from build123d import *

# Parameters (mm, degrees)
SKETCH_1_W          = 26.42
SKETCH_1_H          = 6.6
EXTRUDE_1_DEPTH     = 4.4
SKETCH_2_W          = 12.3
SKETCH_2_H          = 8.6
EXTRUDE_2_DEPTH     = 1.6
SKETCH_3_W          = 4.1
SKETCH_3_H          = 6.6
EXTRUDE_3_DEPTH     = 9.7
FILLET_1_R          = 3
FILLET_2_R          = 1
SKETCH_4_W          = 6
SKETCH_4_H          = 1
EXTRUDE_4_DEPTH     = 1
SKETCH_5_W          = 0.293200104
SKETCH_5_H          = 0.293200104
SKETCH_5_W_2        = 0.377208019
SKETCH_5_W_3        = 0.433090687
EXTRUDE_5_DEPTH     = 1
SKETCH_6_W          = 0.293200104
SKETCH_6_H          = 0.267980564
SKETCH_6_W_2        = 0.377208019
SKETCH_6_W_3        = 0.433090687
EXTRUDE_6_DEPTH     = 6
SKETCH_7_R          = 1.75
CUT_EXTRUDE_1_DEPTH = 6


with BuildPart() as part:
    # 草图1 → 凸台-拉伸1 (new body)
    with BuildSketch(Plane(origin=(0, 0, 0), x_dir=(1, 0, 0), z_dir=(0, 1, 0))):
        with Locations((13.21, 3.3)):
            Rectangle(SKETCH_1_W, SKETCH_1_H)
    extrude(amount=EXTRUDE_1_DEPTH)

    # 草图2 → 凸台-拉伸2 (add)
    with BuildSketch(Plane(origin=(0, 0, 0), x_dir=(-1, 0, 0), z_dir=(0, -1, 0))):
        with Locations((-13.21, -4.3)):
            Rectangle(SKETCH_2_W, SKETCH_2_H)
    extrude(amount=-EXTRUDE_2_DEPTH)

    # 草图3 → 凸台-拉伸3 (add)
    with BuildSketch(Plane(origin=(0, 4.4, 0), x_dir=(1, 0, 0), z_dir=(0, 1, 0))):
        with Locations((8.21, 3.3)):
            Rectangle(SKETCH_3_W, SKETCH_3_H)
        with Locations((18.21, 3.3)):
            Rectangle(SKETCH_3_W, SKETCH_3_H)
    extrude(amount=EXTRUDE_3_DEPTH)

    # 圆角1
    fillet_1_edges = [part.edges().sort_by_distance(p)[0] for p in [
        (0, 2.2, -6.6),
        (26.42, 2.2, -6.6),
        (26.42, 2.2, 0),
        (0, 2.2, 0),
    ]]
    fillet(fillet_1_edges, radius=FILLET_1_R)

    # 圆角2
    fillet_2_edges = [part.edges().sort_by_distance(p)[0] for p in [
        (7.06, 0.8, 8.6),
        (19.36, 0.8, 8.6),
    ]]
    fillet(fillet_2_edges, radius=FILLET_2_R)

    # 草图4 → 凸台-拉伸4 (add)
    with BuildSketch(Plane(origin=(0, 0, 0), x_dir=(-1, 0, 0), z_dir=(0, -1, 0))):
        with Locations((-13.21, -7.5)):
            Rectangle(SKETCH_4_W, SKETCH_4_H)
    extrude(amount=EXTRUDE_4_DEPTH)

    # 草图5 → 凸台-拉伸5 (add)
    with BuildSketch(Plane(origin=(0, -1, 0), x_dir=(-1, 0, 0), z_dir=(0, -1, 0))):
        with Locations((-11.206465954, -7.438185624)):
            Rectangle(SKETCH_5_W, SKETCH_5_H)
        with Locations((-13.359332723, -7.438185624)):
            Rectangle(SKETCH_5_W_2, SKETCH_5_H)
        with Locations((-15.259343482, -7.438185624)):
            Rectangle(SKETCH_5_W_3, SKETCH_5_H)
    extrude(amount=EXTRUDE_5_DEPTH)

    # 草图6 → 凸台-拉伸6 (add)
    with BuildSketch(Plane.XY.offset(7.584785676)):
        with Locations((11.206465954, -1.866009718)):
            Rectangle(SKETCH_6_W, SKETCH_6_H)
        with Locations((13.359332723, -1.866009718)):
            Rectangle(SKETCH_6_W_2, SKETCH_6_H)
        with Locations((15.259343482, -1.866009718)):
            Rectangle(SKETCH_6_W_3, SKETCH_6_H)
    extrude(amount=EXTRUDE_6_DEPTH)

    # 草图7 → 切除-拉伸1 (cut)
    with BuildSketch(Plane(origin=(0, 4.4, 0), x_dir=(1, 0, 0), z_dir=(0, 1, 0))):
        with Locations(Location((2.8, 3.3, 0), (0, 0, 270))):
            Circle(SKETCH_7_R)
        with Locations(Location((23.62, 3.3, 0), (0, 0, 270))):
            Circle(SKETCH_7_R)
    extrude(amount=-CUT_EXTRUDE_1_DEPTH, mode=Mode.SUBTRACT)


solid = part.part
Part model, mm, in its own coordinate system. A direction names the side the tool comes from. Coordinates: 2 decimals unless noted, no trailing zeros. Loops run counter-clockwise (first coordinate to the right, second up) from the corner with the lowest first, then second, coordinate; pieces in that order, holes last. Notation, with made-up numbers: M -14,34.25 L 39,34.25 A21 cw 39,72.25 Z; hole C 40.25,-6.75 d5. An arc over 180 degrees is marked long. Use a Markdown table: item, result. Add a question column.
Q1. Which spindle directions (+Z, -Z, +X, -X, +Y, -Y) get a long thin tool onto all of the face, cutting with end or side? Do faces 4 (the flat face through (10.21, -0.5, 7.5)), 5 (the flat face through (13.3, -0.5, 7)), 6 (the flat face through (13, 1.6, 4)), 7 (the flat face through (10.26, 9, -3)), 8 (the flat face through (21, 4.4, -3)). Say none if no direction does.
Q2. Pin check, flat tips, straight feed: P1, Ø5.5, axis at y = 11, z = -4, coming from the -X side; P2, Ø8, axis at y = 0.5, z = 7, coming from the -X side; P3, Ø3, axis at x = 14.5, y = 1.5, coming from the +Z side. Stop position of each tip, or through.
Q3. Cut at D-D (x = 3.5). Write the cut outline in (y, z).
Q4. Mould opens along X. For faces 1 (the flat face through (16.21, -0.5, 7.5)), 2 (the flat face through (13, 4.4, -3)), 3 (the flat face through (13.3, -0.5, 8)) say: +X half, -X half, draft (parallel to the pull), parting line (faces both ways), or undercut.
Q5. Cut at B-B (z = -3.3). Write the cut outline in (x, y).
Q6. Cut at C-C (y = 9). Write the cut outline in (x, z).
Q7. Probe L1, parallel to X at y = 1.85, z = -3.3; L2, parallel to X at y = 7.75, z = -3; L3, parallel to Y at x = 19, z = 8. List the from-to ranges inside material, lowest first.
Q8. Cut at A-A (y = 0.5). Write the cut outline in (x, z), and give its area (3 significant figures).
Worked out:
| question | item | result |
|---|---|---|
| 1 | face 4 | +Z, -Z, -X, -Y |
| 1 | face 5 | -Z, +X, -X, -Y |
| 1 | face 6 | +Z, +X, -X, +Y |
| 1 | face 7 | +Z, -Z, +Y |
| 1 | face 8 | +Z, -Z, +X, +Y |
| 2 | P1 | stops at x = 6.16 |
| 2 | P2 | stops at x = 7.06 |
| 2 | P3 | stops at z = 8.6 |
| 3 | outline | M 0,-6.6 L 4.4,-6.6 L 4.4,-4.9 L 0,-4.9 Z; M 0,-1.7 L 4.4,-1.7 L 4.4,0 L 0,0 Z |
| 4 | face 1 | +X half |
| 4 | face 2 | undercut |
| 4 | face 3 | draft |
| 5 | outline | M 0,0 L 1.05,0 L 1.05,4.4 L 0,4.4 Z; M 4.55,0 L 21.87,0 L 21.87,4.4 L 20.26,4.4 L 20.26,14.1 L 16.16,14.1 L 16.16,4.4 L 10.26,4.4 L 10.26,14.1 L 6.16,14.1 L 6.16,4.4 L 4.55,4.4 Z; M 25.37,0 L 26.42,0 L 26.42,4.4 L 25.37,4.4 Z |
| 6 | outline | M 6.16,-6.6 L 10.26,-6.6 L 10.26,0 L 6.16,0 Z; M 16.16,-6.6 L 20.26,-6.6 L 20.26,0 L 16.16,0 Z |
| 7 | L1 | x = 0 to 1.05, 4.55 to 21.87, 25.37 to 26.42 |
| 7 | L2 | x = 6.16 to 10.26, 16.16 to 20.26 |
| 7 | L3 | y = 0 to 1.6 |
| 8 | outline | M 0,-3.6 A3 ccw 3,-6.6 L 23.42,-6.6 A3 ccw 26.42,-3.6 L 26.42,-3 A3 ccw 23.42,0 L 19.36,0 L 19.36,7.6 A1 ccw 18.36,8.6 L 8.06,8.6 A1 ccw 7.06,7.6 L 7.06,0 L 3,0 A3 ccw 0,-3 Z; hole C 2.8,-3.3 d3.5; hole C 23.62,-3.3 d3.5 |
| 8 | area | 253 mm2 |
